Input: part model. Units: mm. Frame: model coordinates. Face numbers are marked on the shaded views. A direction names the side the tool comes from. Coordinates: 2 decimals unless noted, no trailing zeros. Write each loop counter-clockwise with the first axis right and the second up, starting at its lowest first coordinate (ties: lowest second). Pieces come first, ordered by that corner, then holes. Notation, with made-up numbers: (-10.5, -24) - (40.5, -24) arc R21 ccw to (40.5, 10) - close; hole circle Ø9 at (-26.75, 53). An arc over 180 degrees is marked (long way). One line per question, with ' | ' between items. Start each with the question number.
1) First-contact query: P1, Ø4, axis at x = 10, z = 24, coming from the -Y side; P2, Ø2, axis at x = 19.5, z = 24.5, coming from the -Y side; P3, Ø3, axis at y = 25, z = 18.5, coming from the -X side. Flat tips, straight axial feed; report the tip coordinate or a pass-through.
2) Reachability of the marked faces 1 and 2 from +Z, -Z, +X, -X, +Y, -Y: full face, straight path, thin tool, end or side. Return the list, or none.
3) Section query B-B on x = 16. Return loops of the section in (y, z), and give its area (3 significant figures).
4) Section query C-C on z = 20. Return loops of the section in (x, y), and give its area (3 significant figures).
5) Section query A-A on y = 30. Return loops of the section in (x, z).
6) Section query D-D on z = 29.5. Return loops of the section in (x, y) (3 decimals).
7) Line query: line 1 (Z direction, x = 22.75, y = 25.25); line 2 (Z direction, x = 9.5, y = 33.5); line 3 (Y direction, x = 13.25, z = 22). Output: solid intervals per line, ascending.
```python
from build123d import *

# Parameters (mm, degrees)
CYLINDER_R     = 6.45
CYLINDER_DEPTH = 12.9


with BuildPart() as cone:
    # Cone → Cone (revolve)
    with BuildSketch(Plane.XZ):
        Polygon((0, 0), (8.75, 0), (6, 5), (0, 5), align=None)
    revolve(axis=Axis((0, 0, 0), (0, 0, 1)))


with BuildPart() as button:
    # Cylinder → Cylinder (new body)
    with BuildSketch(Plane.XY.offset(-12.9)):
        Circle(CYLINDER_R)
    extrude(amount=CYLINDER_DEPTH)

    # Fusion: union Cone
    add(cone.part)


with BuildPart() as button_1:
    # Fusion placement: moved
    add(button.part.moved(Location((16, 30, 27))))


solid = button_1.part
```
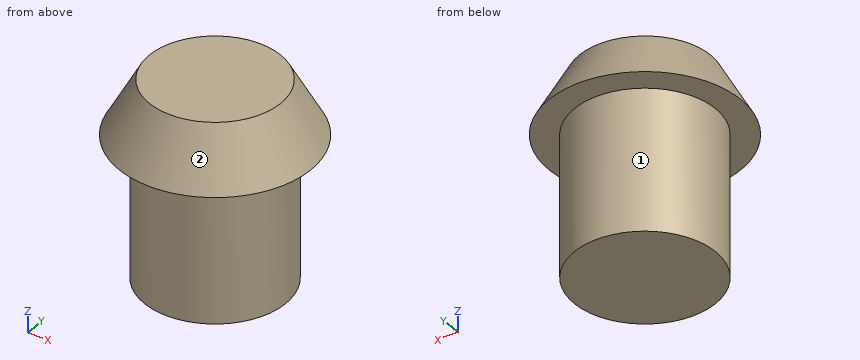
Answer key:
1) P1: y = 24.94 | P2: y = 24.05 | P3: x = 10.58
2) face 1: -Z | face 2: +Z
3) outline: (21.25, 27) - (23.55, 27) - (23.55, 14.1) - (36.45, 14.1) - (36.45, 27) - (38.75, 27) - (36, 32) - (24, 32) - close | area: 240 mm²
4) outline: circle Ø12.9 at (16, 30) | area: 131 mm²
5) outline: (7.25, 27) - (9.55, 27) - (9.55, 14.1) - (22.45, 14.1) - (22.45, 27) - (24.75, 27) - (22, 32) - (10, 32) - close
6) outline: circle Ø14.75 at (16, 30)
7) line 1: 27 to 27.9 | line 2: 27 to 29.49 | line 3: 24.17 to 35.83
